Autodesk Inventor part; units mm, degrees
ref_plane "YZ Plane" through (0, 0, 0) normal (1, 0, 0) x (0, 1, 0)
ref_plane "XZ Plane" through (0, 0, 0) normal (0, 1, 0) x (-1, 0, 0)
ref_plane "XY Plane" through (0, 0, 0) normal (0, 0, 1) x (1, 0, 0)
sketch "Sketch1" plane through (0, 0, 0) normal (0, 0, 1) x (1, 0, 0)
  circle A0 centre (-44.4686, 23.8242) radius 2.5654
  circle A1 centre (44.4314, 23.8242) radius 2.5654
  line L0 (0, 25.1324) -> (0, 21.8881) construction
  circle A2 centre (-44.4686, -23.8008) radius 2.5654
  circle A3 centre (44.4314, -23.8008) radius 2.5654
  line L1 (44.4314, 23.8242) -> (44.4314, -23.8008)
  line L2 (-49.53, -28.575) -> (49.53, -28.575)
  line L3 (49.53, -28.575) -> (49.53, 28.575)
  line L4 (49.53, 28.575) -> (-49.53, 28.575)
  line L5 (-49.53, 28.575) -> (-49.53, -28.575)
  line L6 (-49.53, -28.575) -> (49.53, 28.575) construction
  line L7 (49.53, -28.575) -> (-49.53, 28.575) construction
  point P0 (0, 0)
  dimension "d0" = 5.1308
  dimension "d1" = 5.1308
  dimension "d2" = 88.9
  dimension "d5" = 47.625
  dimension "d10" = 99.06
  dimension "d11" = 57.15
extrude "Extrusion1" add sketch "Sketch1" along normal blind 3.175
fillet "Fillet1" radius 3.175 4 edges at (-49.53, 28.575, 1.5875) (49.53, 28.575, 1.5875) (49.53, -28.575, 1.5875) (-49.53, -28.575, 1.5875)
properties part number "Limelight"
Read the model definition and answer for the solid it produces. Units are mm, in the model's axes. Give positions to 0.01 mm unless a question says otherwise; leave off trailing zeros. Order: outer loops, then holes, each group sorted by start corner. A loop starts at its lowest first (then second) coordinate and runs counter-clockwise, first axis right, second up.
(1) Given pin 1 (3 mm diameter, centred on x = -44.47, y = 23.82, fed in from +Z), flat-ended and moving along its own axis, determine where the tip first touches the part or whether it passes through.
(2) For a pull along Y with two mould halves and no side action, classify faces 1 (the cylindrical face through (-43.09, 21.66, 1.57)), 2 (the cylindrical face through (48.575, -27.67, 1.61)), 3 (the cylindrical face through (-43.089, -25.964, 1.565)), 4 (the flat face through (1, 28.575, 2)) as released by +Y, released by -Y, zero draft, split by the parting line, or undercut.
(3) Find section A-A (x = -44). Give the vertices of the cut face in (y, z) (3 decimals).
(4) Find section B-B (z = 2.25). Give the vertices of the cut face in (x, y) (3 decimals).
Result sheet:
1. pin 1: passes through
2. face 1: undercut
2. face 2: released by -Y
2. face 3: undercut
2. face 4: released by +Y
3. outline: (-28.575, 0) - (-26.323, 0) - (-26.323, 3.175) - (-28.575, 3.175) - close; (-21.279, 0) - (21.302, 0) - (21.302, 3.175) - (-21.279, 3.175) - close; (26.346, 0) - (28.575, 0) - (28.575, 3.175) - (26.346, 3.175) - close
4. outline: (-49.53, -25.4) arc R3.175 ccw to (-46.355, -28.575) - (46.355, -28.575) arc R3.175 ccw to (49.53, -25.4) - (49.53, 25.4) arc R3.175 ccw to (46.355, 28.575) - (-46.355, 28.575) arc R3.175 ccw to (-49.53, 25.4) - close; hole circle Ø5.131 at (-44.469, -23.801); hole circle Ø5.131 at (-44.469, 23.824); hole circle Ø5.131 at (44.431, -23.801); hole circle Ø5.131 at (44.431, 23.824)
